Here's how the part is built. I have some questions about the finished solid (model axes, mm). Face numbers are marked on the shaded views. A direction names the side the tool comes from. Coordinates: 2 decimals unless noted, no trailing zeros. Write each loop counter-clockwise with the first axis right and the second up, starting at its lowest first coordinate (ties: lowest second). Pieces come first, ordered by that corner, then holes.
Item 1: I want a section at B-B (y = -8.75). Please give me the cut outline in (x, z), and give its area (3 significant figures).
Item 2: Please list where these lines run through material, in increasing order: line 1 (Y direction, x = -1.5, z = -4.75); line 2 (Z direction, x = -1.25, y = -10.5); line 3 (Z direction, x = -2, y = -13.75).
Item 3: I want a section at A-A (x = 0). Please give me the cut outline in (y, z).
Item 4: For the marked faces 1 and 2, which set-ups out of +Z, -Z, +X, -X, +Y, -Y let a thin tool reach every point of the face, with its end or its side?
Item 5: I'm going to push flat-ended pins straight in: P1, Ø1, axis at x = -0.5, y = -13, coming from the +Z side; P2, Ø2, axis at x = -4, y = -12.5, coming from the -Z side; P3, Ø4, axis at y = -10.5, z = -2, coming from the -X side. Where does each tip first touch, or does it pass through?
from build123d import *

# Parameters (mm, degrees)
EXTRUDE1_DEPTH = 5.3
SKETCH2_R      = 4
EXTRUDE2_DEPTH = 10


with BuildPart() as part:
    # Sketch1 → Extrude1 (new body)
    with BuildSketch(Plane(origin=(0, 0, 0), x_dir=(1, 0, 0), z_dir=(0, 1, 0))):
        Polygon((7.505553499, 0), (3.75277675, 6.5), (-3.75277675, 6.5), (-7.505553499, 0), (-3.75277675, -6.5), (3.75277675, -6.5), align=None)
    extrude(amount=-EXTRUDE1_DEPTH)

    # Sketch2 → Extrude2 (add)
    with BuildSketch(Plane.XZ.offset(5.3)):
        with Locations(Location((0, 0, 0), (0, 0, 270))):
            Circle(SKETCH2_R)
    extrude(amount=EXTRUDE2_DEPTH)

    # Sketch3 → Cut-Revolve1 (revolve, cut)
    with BuildSketch(Plane.XY):
        Polygon((6.105553499, 0), (7.505553499, 0), (7.505553499, -0.808290377), align=None)
        Polygon((7.505553499, -5.3), (7.505553499, -4.491709623), (6.105553499, -5.3), align=None)
    revolve(axis=Axis((0, -1000, 0), (0, 1, 0)), mode=Mode.SUBTRACT)


solid = part.part
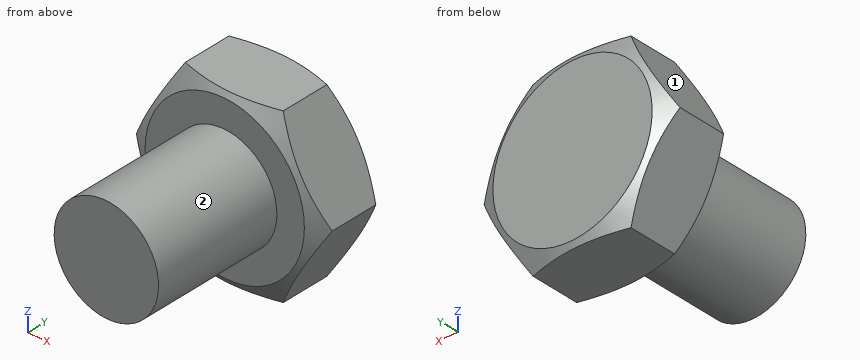
Answer:
1. outline: circle Ø8 at (0, 0)
1. area: 50.3 mm2
2. line 1: y = -5.3 to 0
2. line 2: z = -3.8 to 3.8
2. line 3: z = -3.46 to 3.46
3. outline: (-15.3, -4) - (-5.3, -4) - (-5.3, -6.11) - (-5.07, -6.5) - (-0.23, -6.5) - (0, -6.11) - (0, 6.11) - (-0.23, 6.5) - (-5.07, 6.5) - (-5.3, 6.11) - (-5.3, 4) - (-15.3, 4) - close
4. face 1: +Z, -X, +Y, -Y
4. face 2: -Y
5. P1: stops at z = 4
5. P2: stops at z = -2.65
5. P3: stops at x = -4
